from build123d import *

# Parameters (mm, degrees)
F0_W      = 135
F0_H      = 90
F1_DEPTH  = 20
F2_W      = 55
F2_H      = 14.937833
F3_DEPTH  = 90
F4_W      = 35.29747
F4_H      = 17.323516
F5_DEPTH  = 37
F6_W      = 33.973107
F6_H      = 14.05538
F7_DEPTH  = 47
F9_DEPTH  = 6
F11_DEPTH = 75
F12_R     = 10
F13_DEPTH = 105.001
F14_R     = 6
F15_DEPTH = 10.001
F16_W     = 6
F16_H     = 55
F17_DEPTH = 65
F19_DEPTH = 6


with BuildPart() as f1:
    # F0 (on Top) → F1 (new body)
    with BuildSketch(Plane.XY):
        Rectangle(F0_W, F0_H)
    extrude(amount=F1_DEPTH)

    # F2 (on face) → F3 (cut, through all)
    with BuildSketch(Plane.XZ.offset(45)):
        with Locations((0, 2.531084)):
            Rectangle(F2_W, F2_H)
    extrude(amount=-F3_DEPTH, mode=Mode.SUBTRACT)

    # F4 (on face) → F5 (cut)
    with BuildSketch(Plane.XZ.offset(45)):
        with Locations((-55.148735, 18.661758)):
            Rectangle(F4_W, F4_H)
        with Locations((55.148735, 18.661758)):
            Rectangle(F4_W, F4_H)
    extrude(amount=-F5_DEPTH, mode=Mode.SUBTRACT)

    # F6 (on face) → F7 (cut)
    with BuildSketch(Plane(origin=(0, 45, 0), x_dir=(-1, 0, 0), z_dir=(0, 1, 0))):
        with Locations((-54.486553, 17.02769)):
            Rectangle(F6_W, F6_H)
        with Locations((54.486553, 17.02769)):
            Rectangle(F6_W, F6_H)
    extrude(amount=-F7_DEPTH, mode=Mode.SUBTRACT)

    # F8 (on face) → F9 (cut, through all)
    with BuildSketch(Plane.XZ.offset(8)):
        Polygon((-69.806829, 10), (-67.5, 10), (-37.5, 20), (-37.5, 24.232961), (-69.806829, 24.232961), align=None)
        Polygon((69.806829, 24.232961), (37.5, 24.232961), (37.5, 20), (67.5, 10), (69.806829, 10), align=None)
    extrude(amount=-F9_DEPTH, mode=Mode.SUBTRACT)

    # F10 (on face) → F11 (join, through all)
    with BuildSketch(Plane(origin=(-37.5, 0, 0), x_dir=(0, -1, 0), z_dir=(-1, 0, 0))):
        with BuildLine():
            Line((-45, 65), (-45, 20))
            Line((-45, 20), (-5, 20))
            Line((-5, 20), (-5, 65))
            ThreePointArc((-5, 65), (-25, 85), (-45, 65))
        make_face()
    extrude(amount=-F11_DEPTH)

    # F12 (on face) → F13 (cut, through all)
    with BuildSketch(Plane(origin=(-37.5, 0, 0), x_dir=(0, -1, 0), z_dir=(-1, 0, 0))):
        with Locations((-25, 65)):
            Circle(F12_R)
    extrude(amount=-F13_DEPTH, mode=Mode.SUBTRACT)

    # F14 (on face) → F15 (cut, through all)
    with BuildSketch(Plane.XY.offset(10)):
        with Locations((-52.5, -25)):
            Circle(F14_R)
        with Locations((-52.5, 25)):
            Circle(F14_R)
        with Locations((52.5, -25)):
            Circle(F14_R)
        with Locations((52.5, 25)):
            Circle(F14_R)
    extrude(amount=-F15_DEPTH, mode=Mode.SUBTRACT)

    # F16 (on face) → F17 (join)
    with BuildSketch(Plane.XY.offset(20)):
        with Locations((3, -17.5)):
            Rectangle(F16_W, F16_H)
    extrude(amount=F17_DEPTH)

    # F18 (on face) → F19 (cut)
    with BuildSketch(Plane(origin=(0, 0, 0), x_dir=(0, -1, 0), z_dir=(-1, 0, 0))):
        Polygon((-10, 78.228757), (45, 20), (45, 85), (-10, 85), align=None)
    extrude(amount=-F19_DEPTH, mode=Mode.SUBTRACT)


solid = f1.part
The model under review builds one solid part; all positions refer to its coordinate system, in mm. A direction names the side the tool comes from. Give positions to 0.01 mm unless a question says otherwise; leave off trailing zeros. Loops run counter-clockwise (first coordinate to the right, second up) from the corner with the lowest first, then second, coordinate; pieces in that order, holes last. Notation, with made-up numbers: (37, -1.5) -> (53, -1.5) arc R9 ccw to (53, 11.5) -> close; hole circle Ø10 at (38.25, 82). An arc over 180 degrees is marked (long way). Put each result on its own line as item: value. Start each with the question number.
1. We need section A-A on z = 7.5. State the section outline as (x, y) points, then the cut area to 3 significant figures.
2. Wall thickness on probe 1 along Y at (x, z) = (52.5, 5); probe 2 along X at (y, z) = (-18, 15.5); probe 3 along Z at (x, y) = (60.5, 3.5): over which ranges is each line inside the solid? List them lowest first.
3. Mouldability with a two-part tool opening along X and no side actions: class faces 6 (the face through (-46, -2, 14)), 7 (the face through (-27.5, -1, 5)), 8 (the face through (37.5, -27, 15)) as released by +X, released by -X, zero draft, split by the parting line, or undercut.
4. We need section C-C on y = 25. State the section outline as (x, z) points.
5. We need section D-D on x = 33. State the section outline as (y, z) points.
6. We need section B-B on x = -52.5. State the section outline as (y, z) points.
7. For faces 1 (the face through (46, -2, 13)), 2 (the face through (46, -8, 13)), 3 (the face through (-52, 17, 10)), 4 (the face through (-46, -8, 13)), 5 (the face through (27.5, -1, 5)), list the 3-axis set-ups (+Z, -Z, +X, -X, +Y, -Y) from which the entire face can be reached by the end or side of a thin tool; tool diameter is ignored.
8. Clearance check with flat-ended pins moving along their axes: P1, Ø2, axis at x = 1, z = 74, coming from the +Y side; P2, Ø8, axis at x = -48.5, z = 15, coming from the -Y side; P3, Ø2, axis at x = 9, z = 44, coming from the -Y side; P4, Ø2, axis at x = -29.5, y = -25.5, coming from the -Z side. State where each tip first meets the part, or that it passes through.
Determined:
1. outline: (-67.5, -45) -> (-27.5, -45) -> (-27.5, 45) -> (-67.5, 45) -> close; (27.5, -45) -> (67.5, -45) -> (67.5, 45) -> (27.5, 45) -> close; hole circle Ø12 at (-52.5, -25); hole circle Ø12 at (-52.5, 25); hole circle Ø12 at (52.5, -25); hole circle Ø12 at (52.5, 25)
1. area: 6,750 mm^2
2. probe 1: -45 to -31, -19 to 19, 31 to 45
2. probe 2: -37.5 to 37.5
2. probe 3: 0 to 10
3. face 6: zero draft
3. face 7: undercut
3. face 8: released by +X
4. outline: (-67.5, 0) -> (-58.5, 0) -> (-58.5, 10) -> (-67.5, 10) -> close; (-46.5, 0) -> (-27.5, 0) -> (-27.5, 10) -> (27.5, 10) -> (27.5, 0) -> (46.5, 0) -> (46.5, 10) -> (37.5, 10) -> (37.5, 55) -> (-37.5, 55) -> (-37.5, 10) -> (-46.5, 10) -> close; (-37.5, 75) -> (37.5, 75) -> (37.5, 85) -> (-37.5, 85) -> close; (58.5, 0) -> (67.5, 0) -> (67.5, 10) -> (58.5, 10) -> close
5. outline: (-45, 0) -> (45, 0) -> (45, 65) arc R20 ccw to (5, 65) -> (5, 20) -> (-45, 20) -> close; hole circle Ø20 at (25, 65)
6. outline: (-45, 0) -> (-31, 0) -> (-31, 10) -> (-45, 10) -> close; (-19, 0) -> (19, 0) -> (19, 10) -> (-2, 10) -> (-2, 15) -> (-8, 15) -> (-8, 10) -> (-19, 10) -> close; (31, 0) -> (45, 0) -> (45, 10) -> (31, 10) -> close
7. face 1: +Z, +X, +Y
7. face 2: +Z, +X, -Y
7. face 3: +Z, -X, +Y
7. face 4: +Z, -X, -Y
7. face 5: -Z, +Y, -Y
8. P1: y = 43.33
8. P2: y = -8
8. P3: y = 5
8. P4: z = 0
